Check sheet for the modelled part. Datum: model origin and axes. Units: mm. Give positions to 0.01 mm unless a question says otherwise; leave off trailing zeros. Loops run counter-clockwise (first coordinate to the right, second up) from the corner with the lowest first, then second, coordinate; pieces in that order, holes last. Notation, with made-up numbers: (-29, -3) - (13, -3) arc R26 cw to (13, 12) - close; hole circle Ø4 at (-12.75, 20.25). An arc over 180 degrees is marked (long way). Answer in a Markdown table with one row per item. Add a question column.
(1) Thickness scan on L1, parallel to Y at x = -40, z = 3.1; L2, parallel to Y at x = -12.5, z = 3.8. Record the ranges inside material, lowest first.
(2) Sectioned sample at B-B on z = 3.25. Enter the section's corners in (x, y).
(3) Sectioned sample at C-C on y = 0. Enter the section's corners in (x, z).
(4) Sectioned sample at D-D on x = -85. Enter the section's corners in (y, z).
(5) Sectioned sample at A-A on x = 12.5. Enter the section's corners in (y, z).
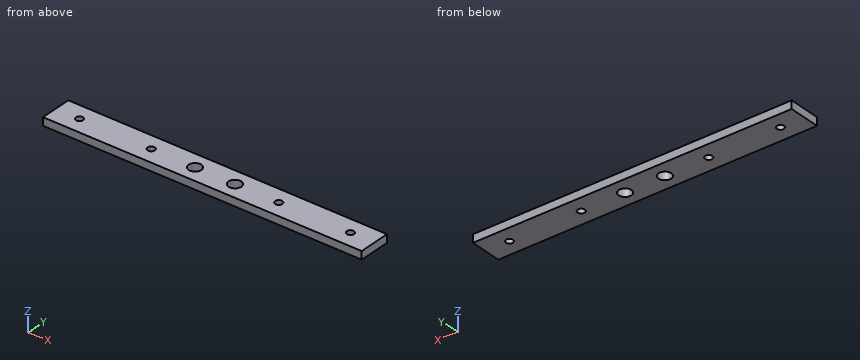
from build123d import *

# Parameters (mm, degrees)
ESQUISSE1_W        = 200
ESQUISSE1_H        = 20
ESQUISSE1_R        = 2.25
ESQUISSE1_R_2      = 4
BOSS_EXTRU_1_DEPTH = 5


with BuildPart() as part:
    # Esquisse1 → Boss.-Extru.1 (new body)
    with BuildSketch(Plane.XY):
        Rectangle(ESQUISSE1_W, ESQUISSE1_H)
        with Locations((-85, 0)):
            Circle(ESQUISSE1_R, mode=Mode.SUBTRACT)
        with Locations((-40, 0)):
            Circle(ESQUISSE1_R, mode=Mode.SUBTRACT)
        with Locations(Location((40, 0, 0), (0, 0, 180))):
            Circle(ESQUISSE1_R, mode=Mode.SUBTRACT)
        with Locations(Location((85, 0, 0), (0, 0, 180))):
            Circle(ESQUISSE1_R, mode=Mode.SUBTRACT)
        with Locations((-12.5, 0)):
            Circle(ESQUISSE1_R_2, mode=Mode.SUBTRACT)
        with Locations(Location((12.5, 0, 0), (0, 0, 180))):
            Circle(ESQUISSE1_R_2, mode=Mode.SUBTRACT)
    extrude(amount=BOSS_EXTRU_1_DEPTH)


solid = part.part
Reply:
| question | item | result |
|---|---|---|
| 1 | L1 | -10 to -2.25, 2.25 to 10 |
| 1 | L2 | -10 to -4, 4 to 10 |
| 2 | outline | (-100, -10) - (100, -10) - (100, 10) - (-100, 10) - close; hole circle Ø4.5 at (-85, 0); hole circle Ø4.5 at (-40, 0); hole circle Ø8 at (-12.5, 0); hole circle Ø8 at (12.5, 0); hole circle Ø4.5 at (40, 0); hole circle Ø4.5 at (85, 0) |
| 3 | outline | (-100, 0) - (-87.25, 0) - (-87.25, 5) - (-100, 5) - close; (-82.75, 0) - (-42.25, 0) - (-42.25, 5) - (-82.75, 5) - close; (-37.75, 0) - (-16.5, 0) - (-16.5, 5) - (-37.75, 5) - close; (-8.5, 0) - (8.5, 0) - (8.5, 5) - (-8.5, 5) - close; (16.5, 0) - (37.75, 0) - (37.75, 5) - (16.5, 5) - close; (42.25, 0) - (82.75, 0) - (82.75, 5) - (42.25, 5) - close; (87.25, 0) - (100, 0) - (100, 5) - (87.25, 5) - close |
| 4 | outline | (-10, 0) - (-2.25, 0) - (-2.25, 5) - (-10, 5) - close; (2.25, 0) - (10, 0) - (10, 5) - (2.25, 5) - close |
| 5 | outline | (-10, 0) - (-4, 0) - (-4, 5) - (-10, 5) - close; (4, 0) - (10, 0) - (10, 5) - (4, 5) - close |
